```python
from build123d import *

# Parameters (mm, degrees)
BOSS_EXTRUDE1_DEPTH = 2.54
SKETCH2_W           = 107.95
SKETCH2_H           = 63.5
CUT_EXTRUDE1_DEPTH  = 226.664855764
CUT_EXTRUDE2_START  = -2.54
CUT_EXTRUDE2_DEPTH  = 2.54
SKETCH4_R           = 4.7625
SKETCH4_R_2         = 6.35
CUT_EXTRUDE3_DEPTH  = 226.66485589


# Read off the part's stored shape, not the designer's step: Cut-Extrude2
with BuildPart() as part:
    # Sketch1 → Boss-Extrude1 (new body)
    with BuildSketch(Plane(origin=(0, 0, 0), x_dir=(1, 0, 0), z_dir=(0, 1, 0))):
        with BuildLine():
            Line((215.9, -14.612459999), (215.9, 36.187540001))
            Line((215.9, 36.187540001), (-215.9, 36.187540001))
            Line((-215.9, 36.187540001), (-215.9, -14.612459999))
            ThreePointArc((-215.9, -14.612459999), (-194.259204241, -52.648965299), (-152.4, -65.412459999))
            Line((-152.4, -65.412459999), (152.4, -65.412459999))
            ThreePointArc((152.4, -65.412459999), (194.259204241, -52.648965299), (215.9, -14.612459999))
        make_face()
    extrude(amount=BOSS_EXTRUDE1_DEPTH)

    # Sketch2 → Cut-Extrude1 (cut, through all)
    with BuildSketch(Plane(origin=(0, 2.54, 0), x_dir=(1, 0, 0), z_dir=(0, 1, 0))):
        with Locations((0, -15.875)):
            Rectangle(SKETCH2_W, SKETCH2_H)
    extrude(amount=-CUT_EXTRUDE1_DEPTH, mode=Mode.SUBTRACT)

    # Cut-Extrude2 outline → Cut-Extrude2 (cut)
    with BuildSketch(Plane(origin=(0, 2.54, 0), x_dir=(1, 0, 0), z_dir=(0, 1, 0)).offset(CUT_EXTRUDE2_START)):
        with BuildLine():
            add(Edge.make_bspline(
                [(-215.899999994, 4.835115527), (-215.566109371, 4.600913161), (-214.20332449, 3.575815014), (-211.81883724, 1.254885046), (-208.930212321, -2.798021616), (-206.463783195, -7.807066224), (-204.667192604, -13.474398824), (-203.719076257, -19.343595697), (-203.665482888, -24.926688771), (-204.419435916, -29.846217321), (-205.817811739, -33.905445303), (-207.110427717, -36.090029013), (-207.840384867, -37.055481676), (-207.892164085, -37.122761751)],
                knots=[0.114839475, 0.114839475, 0.114839475, 0.114839475, 0.125, 0.15625, 0.1875, 0.21875, 0.25, 0.28125, 0.3125, 0.34375, 0.375, 0.40625, 0.408621758, 0.408621758, 0.408621758, 0.408621758], degree=3))
            Line((-215.899999994, 4.835115527), (-215.9, -14.612459999))
            ThreePointArc((-215.9, -14.612459999), (-213.044051445, -26.27599059), (-207.892164085, -37.122761751))
        make_face()
        with BuildLine():
            add(Edge.make_bspline(
                [(207.868044886, -37.162504966), (207.809793398, -37.087410994), (207.071460176, -36.116522204), (205.76942942, -33.924763186), (204.364219868, -29.86852613), (203.602011314, -24.951147017), (203.646262202, -19.369088999), (204.584578872, -13.499601085), (206.371728131, -7.830613162), (208.829838854, -2.818725142), (211.711764265, 1.237884913), (214.130027538, 3.598772476), (215.528958726, 4.645764848), (215.899999994, 4.902596054)],
                knots=[0.09109108, 0.09109108, 0.09109108, 0.09109108, 0.09375, 0.125, 0.15625, 0.1875, 0.21875, 0.25, 0.28125, 0.3125, 0.34375, 0.375, 0.386307936, 0.386307936, 0.386307936, 0.386307936], degree=3))
            ThreePointArc((207.868044886, -37.162504966), (213.03625635, -26.297889248), (215.9, -14.612459999))
            Line((215.9, -14.612459999), (215.899999994, 4.902596054))
        make_face()
    extrude(amount=CUT_EXTRUDE2_DEPTH, mode=Mode.SUBTRACT)

    # Sketch4 → Cut-Extrude3 (cut, through all)
    with BuildSketch(Plane(origin=(0, 2.54, 0), x_dir=(1, 0, 0), z_dir=(0, 1, 0))):
        with Locations(Location((100.33, -43.822459999, 0), (0, 0, 270))):
            Circle(SKETCH4_R)
        with Locations(Location((140.97, -12.072459999, 0), (0, 0, 270))):
            Circle(SKETCH4_R_2)
        with Locations(Location((140.97, 15.867540001, 0), (0, 0, 270))):
            Circle(SKETCH4_R_2)
        with Locations(Location((176.53, 15.867540001, 0), (0, 0, 270))):
            Circle(SKETCH4_R_2)
        with Locations(Location((-100.33, -43.822459999, 0), (0, 0, 270))):
            Circle(SKETCH4_R)
        with Locations(Location((-171.45, -27.312459999, 0), (0, 0, 270))):
            Circle(SKETCH4_R_2)
        with Locations(Location((-171.45, 10.787540001, 0), (0, 0, 270))):
            Circle(SKETCH4_R_2)
        with Locations(Location((176.53, -12.072459999, 0), (0, 0, 270))):
            Circle(SKETCH4_R_2)
        with BuildLine():
            Line((164.7825, -42.552459999), (155.2575, -42.552459999))
            ThreePointArc((155.2575, -42.552459999), (160.02, -28.264959999), (164.7825, -42.552459999))
        make_face()
        with BuildLine():
            Line((-134.3025, -9.559927161), (-134.3025, -11.337927161))
            Line((-134.3025, -11.337927161), (-137.4775, -11.337927161))
            Line((-137.4775, -11.337927161), (-137.4775, -9.559927161))
            ThreePointArc((-137.4775, -9.559927161), (-135.89, 5.898040001), (-134.3025, -9.559927161))
        make_face()
    extrude(amount=-CUT_EXTRUDE3_DEPTH, mode=Mode.SUBTRACT)


solid = part.part
```
Input: part model. Units: mm. Frame: model coordinates. Give positions to 0.01 mm unless a question says otherwise; leave off trailing zeros. Order: outer loops, then holes, each group sorted by start corner. A loop starts at its lowest first (then second) coordinate and runs counter-clockwise, first axis right, second up. Notation, with made-up numbers: (-20, 50.5) -> (-5, 50.5) arc R26 cw to (-5, 82.5) -> close; hole circle Ø10 at (1.5, 9.5). An arc over 180 degrees is marked (long way). Write each question's results on one line, items separated by ' | '. Start each with the question number.
Item 1: Line query: line 1 (Z direction, x = -135.89, y = 1.9); line 2 (X direction, y = 2.2, z = -14) (3 decimals); line 3 (X direction, y = 1.8, z = 41) (3 decimals). Output: solid intervals per line, ascending.
Item 2: Cut plane C-C on y = 2. Give the number of separate pieces and of enclosed holes in the cut face, then the cut area to 3 significant figures.
Item 3: Cut plane A-A on x = 38.5. Return the cut outline in (y, z) (3 decimals), then the cut area to 3 significant figures.
Item 4: Mould query, pull axis Z, two halves, no side actions, for faces 1 (the cylindrical face through (-184.58, 1.25, 58.95)), 2 (the cylindrical face through (105.05, 1.29, 43.2)), 3 (the flat face through (-3, 0, -20)), 4 (the cylindrical face through (134.77, 1.29, -17.24)). Classes: pulls with the +Z half, pulls with the -Z half, needs draft (parallel to the pull), parting line crosses it, or undercut.
Item 5: Contact query for flat-ended pins moving along their axis: P1, Ø5, axis at x = -82.5, z = 42.5, coming from the -Y side; P2, Ø0.9, axis at y = 1.5, z = 10, coming from the +X side; P3, Ø1.3, axis at x = 65.5, y = 1.5, coming from the +Z side; P4, Ø1.3, axis at y = 0.5, z = 4, coming from the -X side. Output: stop coordinate, or through.
Item 6: Cut plane B-B on x = 140.97. Return the cut outline in (y, z), then the cut area to 3 significant figures.
Established:
1) line 1: -36.19 to -5.9, 11.34 to 65.41 | line 2: -215.9 to -176.927, -165.973 to -53.975, 53.975 to 134.901, 147.039 to 170.461, 182.599 to 215.9 | line 3: -205.328 to -104.166, -96.494 to -53.975, 53.975 to 96.494, 104.166 to 153.696, 166.344 to 205.328
2) separate pieces: 1 | enclosed holes: 11 | area: 33,700 mm^2
3) outline: (0, -36.188) -> (2.54, -36.188) -> (2.54, -15.875) -> (0, -15.875) -> close; (0, 47.625) -> (2.54, 47.625) -> (2.54, 65.412) -> (0, 65.412) -> close | area: 96.8 mm^2
4) face 1: pulls with the +Z half | face 2: undercut | face 3: needs draft | face 4: undercut
5) P1: y = 0 | P2: x = 205.88 | P3: z = 65.41 | P4: x = -208.77
6) outline: (0, -36.19) -> (2.54, -36.19) -> (2.54, -22.22) -> (0, -22.22) -> close; (0, -9.52) -> (2.54, -9.52) -> (2.54, 5.72) -> (0, 5.72) -> close; (0, 18.42) -> (2.54, 18.42) -> (2.54, 65.41) -> (0, 65.41) -> close | area: 194 mm^2
